Autodesk Inventor part; units mm, degrees
ref_plane "YZ Plane" through (0, 0, 0) normal (1, 0, 0) x (0, 1, 0)
ref_plane "XZ Plane" through (0, 0, 0) normal (0, 1, 0) x (-1, 0, 0)
ref_plane "XY Plane" through (0, 0, 0) normal (0, 0, 1) x (1, 0, 0)
sketch "Sketch1" plane through (0, 0, 0) normal (0, 1, 0) x (-1, 0, 0)
  line L0 (0, 0) -> (200, 0)
  line L1 (200, 0) -> (200, -150)
  line L2 (200, -150) -> (0, -150)
  line L3 (0, -150) -> (0, 0)
  dimension "d0" = 150
  dimension "d1" = 200
extrude "Extrusion1" add sketch "Sketch1" along normal blind 100
sketch "Sketch4" plane through (0, 0, 0) normal (1, 0, 0) x (0, 0, -1)
  line L0 (0, 100) -> (0, 0)
  line L1 (0, 100) -> (150, 100)
  line L2 (0, 0) -> (150, 100)
  line L3 (150, 100) -> (0, 100)
extrude "Extrusion3" cut sketch "Sketch4" against normal blind 200
sketch "Sketch5" plane through (0, 0, -150) normal (0, 0, -1) x (-1, 0, 0)
  line L0 (0, 0) -> (0, 100)
  line L1 (200, 0) -> (0, 0)
  line L2 (0, 100) -> (200, 100)
  line L3 (200, 100) -> (200, 0)
  line L4 (200, 0) -> (0, 0)
  line L5 (0, 0) -> (0, 100)
extrude "Extrusion4" add sketch "Sketch5" along normal blind 80
sketch "Sketch6" plane through (0, 0, -230) normal (0, 0, -1) x (-1, 0, 0)
  line L0 (25, 80) -> (175, 80)
  line L1 (175, 80) -> (175, 20)
  line L2 (175, 20) -> (25, 20)
  line L3 (25, 20) -> (25, 80)
  line L4 (0, 0) -> (200, 0)
  line L5 (200, 100) -> (0, 100)
  line L6 (200, 0) -> (200, 100)
  line L7 (0, 100) -> (0, 0)
  dimension "d11" = 150
  dimension "d12" = 60
  dimension "d13" = 20
  dimension "d14" = 25
extrude "Extrusion5" cut sketch "Sketch6" against normal blind 75 contours L0 L1 L2 L3
sketch "Sketch7" plane through (0, 0, -155) normal (0, 0, -1) x (-1, 0, 0)
  line L0 (25, 20) -> (25, 80)
  line L1 (175, 80) -> (175, 20)
  line L2 (25, 20) -> (25, 80)
  line L3 (25, 80) -> (175, 80)
  line L4 (175, 80) -> (175, 20)
  line L5 (175, 20) -> (25, 20)
  line L6 (200, 0) -> (200, 100)
  line L7 (200, 100) -> (0, 100)
  line L8 (0, 100) -> (0, 0)
  line L9 (0, 0) -> (200, 0)
  line L10 (175, 20) -> (25, 20)
  line L11 (25, 80) -> (175, 80)
  line L12 (25, 20) -> (25, 80)
  line L13 (175, 20) -> (25, 20)
  line L14 (175, 80) -> (175, 20)
  line L15 (75, 50) -> (125, 50)
  line L16 (125, 50) -> (125, 20)
  line L17 (125, 20) -> (75, 20)
  line L18 (75, 20) -> (75, 50)
  point P0 (0, 0)
  dimension "d17" = 50
  dimension "d18" = 30
  dimension "d20" = 0
  dimension "d21" = 50
extrude "Extrusion6" cut sketch "Sketch7" against normal up to next contours L18 L15 L16 L5
sketch "Sketch8" plane through (-175, 20, -230) normal (0, 1, 0) x (1, 0, 0)
  line L0 (100, -200) -> (50, -200)
  line L1 (100, -155) -> (100, -200)
  line L2 (50, -200) -> (50, -155)
  line L3 (50, -155) -> (100, -155)
  line L4 (100, -155) -> (100, -200)
  line L5 (100, -200) -> (50, -200)
  line L6 (50, -200) -> (50, -155)
  line L7 (50, -155) -> (100, -155)
  line L8 (175, -80) -> (175, -230)
  line L9 (175, -80) -> (-25, -80)
  line L10 (-25, -230) -> (-25, -80)
  line L11 (175, -230) -> (-25, -230)
  line L12 (90, -200) -> (60, -200)
  line L13 (60, -200) -> (60, -140)
  line L14 (60, -140) -> (90, -140)
  line L15 (90, -140) -> (90, -200)
  dimension "d24" = 30
  dimension "d25" = 60
  dimension "d26" = 0
  dimension "d27" = 10
extrude "Extrusion7" cut sketch "Sketch8" against normal up to next contours L0 L13 L3 L15 | L3 L13 L14 L15
sketch "Sketch9" plane through (0, 0, -230) normal (1, 0, 0) x (0, 0, -1)
  line L0 (0, 100) -> (0, 0)
  circle A0 centre (0, 50) radius 50
  point P0 (-230, 0)
  dimension "d30" = 100
extrude "Extrusion8" cut sketch "Sketch9" against normal blind 20
sketch "Sketch10" plane through (-200, 0, -230) normal (-1, 0, 0) x (0, 0, 1)
  circle A0 centre (0, 50) radius 50
  line L0 (0, 0) -> (0, 100)
  line L1 (230, 0) -> (0, 0)
  dimension "d33" = 100
extrude "Extrusion9" cut sketch "Sketch10" against normal blind 20
sketch "Sketch12" plane through (-180, 0, -230) normal (-1, 0, 0) x (0, 0, 1)
  point P0 (230, 0)
properties part number "Sumobot v1.0"
Source: CAD feature listing. Evaluate the final solid. Frame: model axes, mm. A direction names the side the tool comes from. Round coordinates to 2 decimals unless told otherwise and drop trailing zeros. Loops run counter-clockwise (first coordinate to the right, second up) from the corner with the lowest first, then second, coordinate; pieces in that order, holes last. Notation, with made-up numbers: M -31,-9.5 L 18,-9.5 A35 cw 18,27.5 Z; hole C 5,-20.75 d3. An arc over 180 degrees is marked long. Return JSON: item names as keys, results as strings. Group by question number.
1. Section query A-A on z = -54.5. Output: boundary loops of the cut face in (x, y), and give its area (3 significant figures).
2. Material intervals for line 1 along X through (y, z) = (60, -219.5); line 2 along X through (y, z) = (45, -126); line 3 along Y through (x, z) = (-59, -201.5), sorted ascending. Write a range as from..to.
3. Pin query (flat end, axial travel): pin 1 (1 mm diameter, centred on x = -79.5, y = 63.5, fed in from +Z); pin 2 (25 mm diameter, centred on y = 73, z = -216, fed in from -X); pin 3 (10 mm diameter, centred on x = -103, y = 11.5, fed in from +Z). Return the tip coordinate at first contact, or that it passes through.
4. Section query C-C on z = -99. Output: boundary loops of the cut face in (x, y).
5. Section query D-D on y = 13. Output: boundary loops of the cut face in (x, z).
6. Reachability of faces 1 (the face through (-25, 50, -193)), 2 (the face through (-9.86, 51.099, -180.012)), 3 (the face through (-75, 35, -107)), 4 (the face through (-85, 10, -60)) from +Z, -Z, +X, -X, +Y, -Y: full face, straight path, thin tool, end or side. Return the list, or none.
7. Mould query, pull axis Z, two halves, no side actions, for faces 5 (the face through (-115, 10, -60)), 6 (the face through (-190.14, 48.901, -180.012)), 7 (the face through (-100, 10, -30)), 8 (the face through (-99, 100, -189)). Classes: released by +Z, released by -Z, zero draft, split by the parting line, or undercut.
8. Section query B-B on x = -155. Output: boundary loops of the cut face in (y, z), and give its area (3 significant figures).
Checks:
{
 "1": {"outline": "M -200,0 L -115,0 L -115,20 L -125,20 L -125,36.33 L -200,36.33 Z; M -85,0 L 0,0 L 0,36.33 L -75,36.33 L -75,20 L -85,20 Z", "area": "5,850 mm²"},
 "2": {"line 1": "x = -180..-175, -25..-20", "line 2": "x = -200..-125, -75..0", "line 3": "y = 0..20, 80..100"},
 "3": {"pin 1": "stops at z = -94.5", "pin 2": "stops at x = -180", "pin 3": "stops at z = -9.75"},
 "4": {"outline": "M -200,0 L 0,0 L 0,66 L -200,66 Z; hole M -125,20 L -75,20 L -75,50 L -125,50 Z"},
 "5": {"outline": "M -200,-196.37 L -180,-196.37 L -180,-230 L -20,-230 L -20,-196.37 L 0,-196.37 L 0,-19.5 L -200,-19.5 Z; hole M -115,-90 L -85,-90 L -85,-30 L -115,-30 Z"},
 "6": {"face 1": "-Z", "face 2": "-Z, +X", "face 3": "+Z, -Z", "face 4": "-Y"},
 "7": {"face 5": "undercut", "face 6": "released by -Z", "face 7": "undercut", "face 8": "zero draft"},
 "8": {"outline": "M 0,-230 L 20,-230 L 20,-155 L 80,-155 L 80,-230 L 100,-230 L 100,-150 L 0,0 Z", "area": "11,000 mm²"}
}
